```python
from build123d import *

# Parameters (mm, degrees)
F1_W     = 265
F1_H     = 193.8
F2_DEPTH = 12
F0_W     = 100
F0_H     = 23.8
F0_W_2   = 49
F0_H_2   = 25
F0_W_3   = 75
F0_W_4   = 149
F0_H_3   = 30
F3_DEPTH = 0.8
F4_DEPTH = 4.25
F5_DEPTH = 5.5
F6_R     = 5


with BuildPart() as f2:
    # F1 (on Top) → F2 (new body)
    with BuildSketch(Plane.XY):
        with Locations((-12.5, -3.1)):
            Rectangle(F1_W, F1_H)
    extrude(amount=-F2_DEPTH)

    # F0 (on Top) → F3 (cut)
    with BuildSketch(Plane.XY):
        Polygon((-100, 73.8), (-125, 73.8), (-125, -6.7), (-100, -6.7), (-100, 50), align=None)
        with Locations((-50, 61.9)):
            Rectangle(F0_W, F0_H)
        Polygon((-63, 38), (-88, 38), (-88, -17.5), (-63, -17.5), (-63, 13), align=None)
        with Locations((-38.5, 25.5)):
            Rectangle(F0_W_2, F0_H_2)
        Polygon((58, 27.5), (33, 27.5), (33, -13), (33, -38), (58, -38), align=None)
        with Locations((-4.5, -25.5)):
            Rectangle(F0_W_3, F0_H_2)
        Polygon((100, -80), (100, 25), (70, 25), (70, -50), (70, -80), align=None)
        with Locations((-4.5, -65)):
            Rectangle(F0_W_4, F0_H_3)
    extrude(amount=-F3_DEPTH, mode=Mode.SUBTRACT)

    # F0 (on Top) → F4 (cut)
    with BuildSketch(Plane.XY):
        Polygon((58, 27.5), (33, 27.5), (33, -13), (33, -38), (58, -38), align=None)
        Polygon((-63, 38), (-88, 38), (-88, -17.5), (-63, -17.5), (-63, 13), align=None)
        Polygon((-100, 73.8), (-125, 73.8), (-125, -6.7), (-100, -6.7), (-100, 50), align=None)
    extrude(amount=-F4_DEPTH, mode=Mode.SUBTRACT)

    # F0 (on Top) → F5 (cut)
    with BuildSketch(Plane.XY):
        Polygon((100, -80), (100, 25), (70, 25), (70, -50), (70, -80), align=None)
    extrude(amount=-F5_DEPTH, mode=Mode.SUBTRACT)

    # F6
    f6_edges = [f2.edges().sort_by_distance(p)[0] for p in [
        (-145, -100, -6),
        (120, -100, -6),
        (120, 93.8, -6),
        (-145, 93.8, -6),
    ]]
    fillet(f6_edges, radius=F6_R)


solid = f2.part
```
Read the model definition and answer for the solid it produces. Units are mm, in the model's axes. A direction names the side the tool comes from. Coordinates: 2 decimals unless noted, no trailing zeros. Order: outer loops, then holes, each group sorted by start corner. A loop starts at its lowest first (then second) coordinate and runs counter-clockwise, first axis right, second up. Notation, with made-up numbers: (75, 60) - (116, 60) arc R6 ccw to (116, 71) - close; hole circle Ø10 at (-5, -9.75). An arc over 180 degrees is marked (long way). Answer as a JSON object with one key per item and string values. Group by question number.
Item 1: Flat-ended cylindrical pins translate along their axes: P1, Ø20, axis at x = 3.5, y = -24, coming from the +Z side; P2, Ø9, axis at x = 79, y = -51, coming from the +Z side; P3, Ø12.5, axis at x = -115, y = 25.5, coming from the +Z side. Find the tip coordinate at first contact, or state that the pin passes through.
Item 2: Section B-B (y = 64) is taken. Give the vertices of the cut face in (x, z), plus the area to 3 significant figures.
Item 3: A tool of negligible diameter and unlimited length cuts with its end or side. For faces 1 (the face through (120, -4, -6)), 2 (the face through (85, -27, -5.5)), from which of +Z, -Z, +X, -X, +Y, -Y can it reach the whole face along a straight path? Write none if from no direction.
Item 4: Consider probe 1 along X at (y, z) = (33.5, -1.75); probe 2 along X at (y, z) = (41.5, -2.25); probe 3 along Y at (x, z) = (-115, -3.25). Determine where each line is inside the solid, lowest interval first. Write a range as from..to.
Item 5: Section C-C (x = -56) is taken. Give the vertices of the cut face in (y, z), plus the area to 3 significant figures.
Item 6: Section A-A (x = 6) is taken. Give the vertices of the cut face in (y, z), plus the area to 3 significant figures.
Item 7: Section D-D (y = -2) is taken. Give the vertices of the cut face in (x, z).
Item 8: The mould has two halves that part along X. Classify faces 3 (the face through (-14, -2, 0)), 4 (the face through (100, -28, -3)), 5 (the face through (-76, 11, -4.25)), 6 (the face through (118.57, 92.3, -6.08)): +X half, -X half, draft (parallel to the pull), parting line (faces both ways), or undercut.
Results are:
{
 "1": {"P1": "stops at z = -0.8", "P2": "stops at z = -5.5", "P3": "stops at z = -4.25"},
 "2": {"outline": "(-145, -12) - (120, -12) - (120, 0) - (0, 0) - (0, -0.8) - (-100, -0.8) - (-100, -4.25) - (-125, -4.25) - (-125, 0) - (-145, 0) - close", "area": "2,990 mm^2"},
 "3": {"face 1": "+Z, -Z, +X, +Y, -Y", "face 2": "+Z"},
 "4": {"probe 1": "x = -145..-125, -100..-88, -63..120", "probe 2": "x = -145..-125, -100..120", "probe 3": "y = -100..-6.7, 73.8..93.8"},
 "5": {"outline": "(-100, -12) - (93.8, -12) - (93.8, 0) - (73.8, 0) - (73.8, -0.8) - (50, -0.8) - (50, 0) - (38, 0) - (38, -0.8) - (13, -0.8) - (13, 0) - (-50, 0) - (-50, -0.8) - (-80, -0.8) - (-80, 0) - (-100, 0) - close", "area": "2,260 mm^2"},
 "6": {"outline": "(-100, -12) - (93.8, -12) - (93.8, 0) - (-13, 0) - (-13, -0.8) - (-38, -0.8) - (-38, 0) - (-50, 0) - (-50, -0.8) - (-80, -0.8) - (-80, 0) - (-100, 0) - close", "area": "2,280 mm^2"},
 "7": {"outline": "(-145, -12) - (120, -12) - (120, 0) - (100, 0) - (100, -5.5) - (70, -5.5) - (70, 0) - (58, 0) - (58, -4.25) - (33, -4.25) - (33, 0) - (-63, 0) - (-63, -4.25) - (-88, -4.25) - (-88, 0) - (-100, 0) - (-100, -4.25) - (-125, -4.25) - (-125, 0) - (-145, 0) - close"},
 "8": {"face 3": "draft", "face 4": "undercut", "face 5": "undercut", "face 6": "+X half"}
}
